from build123d import *

# Parameters (mm, degrees)
SKETCH2_W          = 11
SKETCH2_H          = 50
CUT_EXTRUDE1_DEPTH = 2.8


with BuildPart() as part:
    # Sketch2 → Revolve1 (revolve)
    with BuildSketch(Plane(origin=(0, 0, 0), x_dir=(0, 0, -1), z_dir=(1, 0, 0))):
        with Locations((5.5, -360)):
            Rectangle(SKETCH2_W, SKETCH2_H)
    revolve(axis=Axis((0, -385, 0), (0, 1, 0)))

    # Sketch1 → Cut-Extrude1 (cut, symmetric)
    with BuildSketch(Plane(origin=(0, 0, 0), x_dir=(0, 0, -1), z_dir=(1, 0, 0))):
        Polygon((-38.186717683, 609.980512405), (-17.5, -57.391201416), (-7.5, -380), (7.5, -380), (17.5, -57.391201416), (38.186717683, 609.980512405), (38.186717683, 1945.365018378), (-38.186717683, 1945.365018378), align=None)
    extrude(amount=CUT_EXTRUDE1_DEPTH, both=True, mode=Mode.SUBTRACT)

    # Sketch4 → M3 Clearance Hole1 (revolve, cut)
    with BuildSketch(Plane.ZX.offset(-365)):
        Polygon((0, 0), (0, 11), (1.7, 11), (1.7, 0.020977491), (1.725, 0), align=None)
    m3_clearance_hole1 = revolve(axis=Axis((-6.35, -365, 0), (1, 0, 0)), mode=Mode.SUBTRACT)

    # Mirror1: M3 Clearance Hole1 across plane
    add(m3_clearance_hole1.mirror(Plane(origin=(0, 0, 0), x_dir=(0, 0, 1), z_dir=(1, 0, 0))), mode=Mode.SUBTRACT)


solid = part.part
Build history of the part. All positions in model axes, mm. A direction names the side the tool comes from. Coordinates: 2 decimals unless noted, no trailing zeros. Write each loop counter-clockwise with the first axis right and the second up, starting at its lowest first coordinate (ties: lowest second). Pieces come first, ordered by that corner, then holes. Notation, with made-up numbers: (67, 89.5) -> (106, 89.5) arc R10 ccw to (106, 105.5) -> close; hole circle Ø4 at (-25, -23.5). An arc over 180 degrees is marked (long way). Use CSV: the item, a comma, the result in double quotes. Start each with the question number.
Q1. Drill centre lines: probe 1 along Y at (x, z) = (-5.25, 0); probe 2 along X at (y, z) = (-356, 0.5); probe 3 along Y at (x, z) = (-1.25, 0.5). Where is each one in solid material? Low to high.
Q2. Pull direction Z, two halves, no side cores. Call faces 3 (the flat face through (5, -335, 0)), 4 (the cylindrical face through (10.74, -359.65, 2.38)), 5 (the cylindrical face through (-6.843, -366.686, -0.221)): released by +Z, released by -Z, zero draft, split by the parting line, or undercut.
Q3. Cut at B-B, the plane y = -365. List the corners of the cut face in (x, z), then the cut area to 3 significant figures.
Q4. 3-axis set-ups, long thin cutter, end or side, ignore diameter. For faces 1 (the flat face through (0, -385, 0)), 2 (the flat face through (0, -380, 0)): which of +Z, -Z, +X, -X, +Y, -Y reach the whole face in a straight line?
Q5. Cut at C-C, the plane x = 0. List the corners of the cut face in (y, z).
Q6. Cut at A-A, the plane z = 0. List the corners of the cut face in (x, y).
Q7. Flat gauge pins, fed straight in: pin 1 Ø2 at (y, z) = (-361.5, -2) entering from -X; pin 2 Ø6 at (x, y) = (-9, -344) entering from +Z; pin 3 Ø1.5 at (x, y) = (-6, -356) entering from +Z. Where does each tip first touch, or does it go through?
Q8. Cut at D-D, the plane z = 8. List the corners of the cut face in (x, y).
Checked values:
1,probe 1,"y = -385 to -366.7, -363.3 to -335"
1,probe 2,"x = -10.99 to -2.8, 2.8 to 10.99"
1,probe 3,"y = -385 to -380"
2,face 3,"zero draft"
2,face 4,"split by the parting line"
2,face 5,"undercut"
3,outline,"(-10.87, -1.7) arc R11 ccw to (10.87, -1.7) -> (2.8, -1.7) -> (2.8, -7.96) -> (-2.8, -7.96) -> (-2.8, -1.7) -> close; (-10.87, 1.7) -> (-2.8, 1.7) -> (-2.8, 7.96) -> (2.8, 7.96) -> (2.8, 1.7) -> (10.87, 1.7) arc R11 ccw to start"
3,area,"235 mm²"
4,face 1,"+Z, -Z, +X, -X, -Y"
4,face 2,"+Y"
5,outline,"(-385, -11) -> (-335, -11) -> (-335, -8.89) -> (-380, -7.5) -> (-380, 7.5) -> (-335, 8.89) -> (-335, 11) -> (-385, 11) -> close"
6,outline,"(-11, -385) -> (11, -385) -> (11, -366.7) -> (2.8, -366.7) -> (2.8, -380) -> (-2.8, -380) -> (-2.8, -366.7) -> (-11, -366.7) -> close; (-11, -363.3) -> (-2.8, -363.3) -> (-2.8, -335) -> (-11, -335) -> close; (2.8, -363.3) -> (11, -363.3) -> (11, -335) -> (2.8, -335) -> close"
7,pin 1,"stops at x = -10.95"
7,pin 2,"stops at z = 9.22"
7,pin 3,"stops at z = 9.67"
8,outline,"(-7.55, -385) -> (7.55, -385) -> (7.55, -335) -> (2.8, -335) -> (2.8, -363.87) -> (-2.8, -363.87) -> (-2.8, -335) -> (-7.55, -335) -> close"
